```python
from build123d import *

# Parameters (mm, degrees)
SKETCH_R              = 3.05
PAD_DEPTH             = 7
PAD_DEPTH_BACK        = 10
SKETCH001_R           = 1.05
POCKET_DEPTH          = 5
FILLET_R              = 0.5
CLONE_ROLL_ANGLE      = -0.195955
CLONE_PITCH_ANGLE     = -1.083793
CLONE_PLACEMENT_ANGLE = -0.025657


with BuildPart() as part:
    # Sketch → Pad (new body, two sides)
    with BuildSketch(Plane.XZ) as pad_sk:
        with BuildLine():
            Line((10, 0), (10, -5))
            Line((10, -5), (-10, -5))
            Line((-10, -5), (-10, 0))
            Line((-10, 0), (-5, 0))
            ThreePointArc((5, 0), (0, 5), (-5, 0))
            Line((10, 0), (5, 0))
        make_face()
        Circle(SKETCH_R, mode=Mode.SUBTRACT)
    extrude(amount=PAD_DEPTH)
    extrude(pad_sk.sketch, amount=-PAD_DEPTH_BACK)

    # Sketch001 → Pocket (cut)
    with BuildSketch(Plane(origin=(0, 0, -5), x_dir=(1, 0, 0), z_dir=(0, 0, -1))):
        with Locations((-7.5, 4.5)):
            Circle(SKETCH001_R)
        with Locations((-7.5, -7.5)):
            Circle(SKETCH001_R)
        with Locations((7.5, -7.5)):
            Circle(SKETCH001_R)
        with Locations((7.5, 4.5)):
            Circle(SKETCH001_R)
    extrude(amount=-POCKET_DEPTH, mode=Mode.SUBTRACT)

    # Fillet
    fillet_edges = [part.edges().sort_by_distance(p)[0] for p in [
        (-3.05, 10, 0),
        (-3.05, -7, 0),
    ]]
    fillet(fillet_edges, radius=FILLET_R)


with BuildPart() as part_1:
    # Clone roll: moved
    add(part.part.rotate(Axis((0, 0, 0), (1, 0, 0)), CLONE_ROLL_ANGLE))


with BuildPart() as part_2:
    # Clone pitch: moved
    add(part_1.part.rotate(Axis((0, 0, 0), (0, 1, 0)), CLONE_PITCH_ANGLE))


with BuildPart() as part_3:
    # Clone placement: moved
    add(part_2.part.moved(Location((42.49284, -0.017909, 0.256585))).rotate(Axis((42.49284, -0.017909, 0.256585), (0, 0, 1)), CLONE_PLACEMENT_ANGLE))


solid = part_3.part
```
Could you check a few things on this model? Use its own coordinates, in mm. Coordinates: 2 decimals unless noted, no trailing zeros. Use one line per item in the form item = value. Start each with the question number.
1. Please list where these lines run through material, in increasing order: line 1 (Y direction, x = 34.75, z = -3.5); line 2 (Z direction, x = 41, y = 9); line 3 (Z direction, x = 44.25, y = 2.75).
2. Suppose I cut it at A-A on y = 7. Count the separate pieces of the cut face and the enclosed holes in it, then the cut area to 3 significant figures.
3. For pin 1 (6 mm diameter, centred on x = 35, y = 1.5, fed in from -Z); pin 2 (1.5 mm diameter, centred on x = 48.5, y = -3.5, fed in from -Z); pin 3 (1.5 mm diameter, centred on x = 39, z = -1, fed in from -Y), each with a flat end and sliding along its axis, tell me the tip position at first contact or that it passes through.
Geometry says:
q1.line_1 = -7.03 to -5.53, -3.52 to 6.47, 8.47 to 9.97
q1.line_2 = -4.8 to -2.43, 2.88 to 5
q1.line_3 = -4.72 to -2.25, 2.74 to 4.93
q2.separate_pieces = 3
q2.enclosed_holes = 1
q2.area = 91.3 mm^2
q3.pin_1 = -4.94
q3.pin_2 = -4.63
q3.pin_3 = -7.02
